The listing builds one solid part. Answer for the finished solid, in the listing's coordinates (mm). Give positions to 0.01 mm unless a question says otherwise; leave off trailing zeros. Order: outer loops, then holes, each group sorted by start corner. A loop starts at its lowest first (then second) coordinate and runs counter-clockwise, first axis right, second up. Notation, with made-up numbers: (71, 1) - (93, 1) arc R14 ccw to (93, 10) - close; hole circle Ø1 at (72.25, -33.5). An arc over 180 degrees is marked (long way). Write each question's results on one line, items separated by ' | '. Start each with the question number.
1. Section A-A (x = 1.9) is taken. Give the vertices of the cut face in (y, z), and give its area (3 significant figures).
2. Determine the mould class of faces 1 (the face through (0, -69, -62)), 2 (the face through (1, -140, -50)), 3 (the face through (1.52, -133.71, -4.83)) for opening direction Y: released by +Y, released by -Y, zero draft, split by the parting line, or undercut.
3. Find the intervals of material crossed by L1, parallel to Z at x = 1.95, y = -135; L2, parallel to Y at x = 1.6, z = -97; L3, parallel to Y at x = 2.75, z = -6, in increasing order.
4. Section B-B (y = -75) is taken. Give the vertices of the cut face in (x, z) (3 decimals), and give its area (3 significant figures).
from build123d import *

# Parameters (mm, degrees)
SKETCH1_W           = 102
SKETCH1_H           = 140
BOSS_EXTRUDE1_DEPTH = 3
FILLET1_R           = 5
CUT_EXTRUDE1_DEPTH  = 3
SKETCH3_R           = 1.3
CUT_EXTRUDE2_DEPTH  = 100


with BuildPart() as part:
    # Sketch1 → Boss-Extrude1 (new body)
    with BuildSketch(Plane(origin=(0, 0, 0), x_dir=(0, 0, -1), z_dir=(1, 0, 0))):
        with Locations((51, -70)):
            Rectangle(SKETCH1_W, SKETCH1_H)
    extrude(amount=BOSS_EXTRUDE1_DEPTH)

    # Fillet1
    fillet1_edges = [part.edges().sort_by_distance(p)[0] for p in [
        (1.5, 0, 0),
        (1.5, 0, -102),
        (1.5, -140, -102),
        (1.5, -140, 0),
    ]]
    fillet(fillet1_edges, radius=FILLET1_R)

    # Sketch2 → Cut-Extrude1 (cut)
    with BuildSketch(Plane(origin=(3, 0, 0), x_dir=(0, 0, -1), z_dir=(1, 0, 0))):
        with BuildLine():
            ThreePointArc((46.313735132, -76.483742869), (51, -78), (55.686264868, -76.483742869))
            Line((55.686264868, -76.483742869), (51, -70))
            Line((51, -70), (46.313735132, -76.483742869))
        make_face()
        with BuildLine():
            Line((51, -70), (55.686264868, -76.483742869))
            ThreePointArc((55.686264868, -76.483742869), (58.123556659, -73.640733515), (59, -70))
            ThreePointArc((59, -70), (58.123556659, -66.359266485), (55.686264868, -63.516257131))
            Line((55.686264868, -63.516257131), (51, -70))
        make_face()
        with BuildLine():
            Line((46.313735132, -76.483742869), (51, -70))
            Line((51, -70), (46.313735132, -63.516257131))
            ThreePointArc((46.313735132, -63.516257131), (43, -70), (46.313735132, -76.483742869))
        make_face()
        with BuildLine():
            Line((46.313735132, -63.516257131), (51, -70))
            Line((51, -70), (55.686264868, -63.516257131))
            ThreePointArc((55.686264868, -63.516257131), (51, -62), (46.313735132, -63.516257131))
        make_face()
    extrude(amount=-CUT_EXTRUDE1_DEPTH, mode=Mode.SUBTRACT)

    # Sketch3 → Cut-Extrude2 (cut)
    with BuildSketch(Plane(origin=(3, 0, 0), x_dir=(0, 0, -1), z_dir=(1, 0, 0))):
        with Locations((5, -135)):
            Circle(SKETCH3_R)
        with Locations((5, -5)):
            Circle(SKETCH3_R)
        with Locations((97, -5)):
            Circle(SKETCH3_R)
        with Locations((97, -135)):
            Circle(SKETCH3_R)
    extrude(amount=-CUT_EXTRUDE2_DEPTH, mode=Mode.SUBTRACT)


solid = part.part
Reported:
1) outline: (-140, -97) arc R5 ccw to (-135, -102) - (-5, -102) arc R5 ccw to (0, -97) - (0, -5) arc R5 ccw to (-5, 0) - (-135, 0) arc R5 ccw to (-140, -5) - close; hole circle Ø2.6 at (-135, -97); hole circle Ø2.6 at (-135, -5); hole circle Ø16 at (-70, -51); hole circle Ø2.6 at (-5, -97); hole circle Ø2.6 at (-5, -5) | area: 14,000 mm²
2) face 1: zero draft | face 2: released by -Y | face 3: undercut
3) L1: -102 to -98.3, -95.7 to -6.3, -3.7 to 0 | L2: -140 to -136.3, -133.7 to -6.3, -3.7 to 0 | L3: -140 to -135.83, -134.17 to -5.83, -4.17 to 0
4) outline: (0, -102) - (3, -102) - (3, -57.245) - (0, -57.245) - close; (0, -44.755) - (3, -44.755) - (3, 0) - (0, 0) - close | area: 269 mm²
